```python
from build123d import *

# Parameters (mm, degrees)
F2_W     = 34
F2_H     = 34
F3_DEPTH = 10
F1_W     = 24
F1_H     = 24
F4_DEPTH = 1
F0_W     = 18.5
F0_H     = 18.5
F5_DEPTH = 8
F6_W     = 18.5
F6_H     = 3
F7_DEPTH = 34


with BuildPart() as f3:
    # F2 (on Top) → F3 (new body)
    with BuildSketch(Plane.XY):
        Rectangle(F2_W, F2_H)
    extrude(amount=-F3_DEPTH)

    # F1 (on Top) → F4 (cut)
    with BuildSketch(Plane.XY):
        Rectangle(F1_W, F1_H)
    extrude(amount=-F4_DEPTH, mode=Mode.SUBTRACT)

    # F0 (on Top) → F5 (cut)
    with BuildSketch(Plane.XY):
        Rectangle(F0_W, F0_H)
    extrude(amount=-F5_DEPTH, mode=Mode.SUBTRACT)

    # F6 (on face) → F7 (cut)
    with BuildSketch(Plane.YZ.offset(17)):
        with Locations((0.064, -6.5)):
            Rectangle(F6_W, F6_H)
    extrude(amount=-F7_DEPTH, mode=Mode.SUBTRACT)


solid = f3.part
```
Can you work these out from the model? Positions are in its coordinate system, mm. A direction names the side the tool comes from. Give positions to 0.01 mm unless a question says otherwise; leave off trailing zeros. Order: outer loops, then holes, each group sorted by start corner. A loop starts at its lowest first (then second) coordinate and runs counter-clockwise, first axis right, second up. Notation, with made-up numbers: M 74.5,73 L 132.5,73 A10 cw 132.5,89 Z; hole C 52,27 d2. An arc over 180 degrees is marked long. Write item = value, one per line. Start each with the question number.
Q1. Suppose I cut it at D-D (x = -3). Write out the boundary of the cut face in (y, z).
Q2. Suppose I cut it at C-C (z = -2.5). Write out the boundary of the cut face in (x, y), plus the area to 3 significant figures.
Q3. Suppose I cut it at A-A (y = -1). Write out the boundary of the cut face in (x, z).
Q4. For faces 1 (the flat face through (17, 0, -4)), 2 (the flat face through (-0.2, -12, -0.5)), 3 (the flat face through (0, 9.314, -7)), which set-ups out of +Z, -Z, +X, -X, +Y, -Y let a thin tool reach every point of the face, with its end or its side?
Q5. We'd pull the mould along X, two halves only. Please class faces 4 (the flat face through (12, -0.2, -0.5)), 5 (the flat face through (-17, 0, -4)), 6 (the flat face through (13, -9.186, -7)), 7 (the flat face through (0, -9.25, -4)): pulls with the +X half, pulls with the -X half, needs draft (parallel to the pull), parting line crosses it, or undercut.
Q6. Will this pin go through, and if not, where does the flat tip stop? pin 1 Ø5.5 at (x, y) = (1, -2) entering from +Z.
Q7. I need wall thicknesses on probe 1 along X at (y, z) = (-5, -0.75); probe 2 along X at (y, z) = (1, -4.75); probe 3 along Z at (x, y) = (13.5, -7). Which ranges of each line are inside material? Lowest first, please. Write a range as [from, to].
Q8. Suppose I cut it at B-B (x = 11). Write out the boundary of the cut face in (y, z), plus the area to 4 significant figures.
Check result:
q1.outline = M -17,-10 L 17,-10 L 17,0 L 12,0 L 12,-1 L 9.25,-1 L 9.25,-5 L 9.31,-5 L 9.31,-8 L -9.25,-8 L -9.25,-1 L -12,-1 L -12,0 L -17,0 Z
q2.outline = M -17,-17 L 17,-17 L 17,17 L -17,17 Z; hole M -9.25,-9.25 L 9.25,-9.25 L 9.25,9.25 L -9.25,9.25 Z
q2.area = 814 mm2
q3.outline = M -17,-10 L 17,-10 L 17,-8 L -17,-8 Z; M -17,-5 L -9.25,-5 L -9.25,-1 L -12,-1 L -12,0 L -17,0 Z; M 9.25,-5 L 17,-5 L 17,0 L 12,0 L 12,-1 L 9.25,-1 Z
q4.face_1 = +Z, -Z, +X, +Y, -Y
q4.face_2 = +Z
q4.face_3 = +X, -X
q5.face_4 = undercut
q5.face_5 = pulls with the -X half
q5.face_6 = needs draft
q5.face_7 = undercut
q6.pin_1 = -8
q7.probe_1 = [-17, -12], [12, 17]
q7.probe_2 = [-17, -9.25], [9.25, 17]
q7.probe_3 = [-10, -8], [-5, 0]
q8.outline = M -17,-10 L 17,-10 L 17,0 L 12,0 L 12,-1 L -12,-1 L -12,0 L -17,0 Z; hole M -9.19,-8 L 9.31,-8 L 9.31,-5 L -9.19,-5 Z
q8.area = 260.5 mm2
